Input: part model. Units: mm. Frame: model coordinates. A direction names the side the tool comes from. Coordinates: 2 decimals unless noted, no trailing zeros. Write each loop counter-clockwise with the first axis right and the second up, starting at its lowest first coordinate (ties: lowest second). Pieces come first, ordered by that corner, then holes. Notation, with made-up numbers: (-14, 59.5) - (3, 59.5) arc R16 cw to (3, 73.5) - close; hole circle Ø5 at (-6.5, 88). An arc over 180 degrees is marked (long way). One line per question, with ' | ' between items. Start each with the question number.
1) Section query D-D on x = -15. Return loops of the section in (y, z), and give its area (3 significant figures).
2) First-contact query: P1, Ø2, axis at x = -7, z = 2.5, coming from the +Y side; P2, Ø1.3, axis at x = 4.5, y = 19, coming from the -Z side; P3, Ø1.5, axis at x = 0, z = -0.5, coming from the -Y side; P4, Ø3, axis at y = -8, z = 1, coming from the +X side. Flat tips, straight axial feed; report the tip coordinate or a pass-through.
3) Section query B-B on y = -4.5. Return loops of the section in (x, z).
4) Section query A-A on x = 12.5. Return loops of the section in (y, z), and give its area (3 significant figures).
5) Draft query along Y for faces 4 (the flat face through (0, -15.24, 0)), 5 (the flat face through (-10.16, -17, 0)), 6 (the flat face through (8.924, -7, 0)). Return one class per face: released by +Y, released by -Y, zero draft, split by the parting line, or undercut.
6) Reachability of faces 1 (the flat face through (-19, 9.906, 0)), 2 (the flat face through (0, -17, 2.54)), 3 (the flat face through (3.43, 2.72, 0.07)) from +Z, -Z, +X, -X, +Y, -Y: full face, straight path, thin tool, end or side. Return the list, or none.
7) Line query: line 1 (Y direction, x = 11, z = -2); line 2 (Z direction, x = 15.5, y = 0.5); line 3 (X direction, y = 10, z = 4.75). Output: solid intervals per line, ascending.
8) Section query C-C on x = 8. Return loops of the section in (y, z), and give its area (3 significant figures).
```python
from build123d import *

# Parameters (mm, degrees)
F0_W     = 35.56
F0_H     = 35.56
F1_DEPTH = 5.08
F2_W     = 19.812
F2_H     = 4.572
F3_DEPTH = 2.54
F4_W     = 19.812
F4_H     = 4.572
F5_DEPTH = 2.54
F6_W     = 20.32
F6_H     = 5.08
F7_DEPTH = 2.54
F8_W     = 20.32
F8_H     = 5.08
F9_DEPTH = 2.54


with BuildPart() as f1:
    # F0 (on Top) → F1 (new body, symmetric)
    with BuildSketch(Plane.XY):
        Rectangle(F0_W, F0_H)
        with BuildLine():
            Line((2.5355902778, -12.7), (-2.3592013889, -12.7))
            Line((-2.3592013889, -12.7), (-8.4225694444, 7.0555555556))
            Line((-8.4225694444, 7.0555555556), (-8.5769097222, 7.0555555556))
            add(Edge.make_bspline(
                [(-8.5769097222, 7.0555555556), (-8.2461805556, 1.0307725694), (-8.2461805556, -0.9866753472)],
                knots=[0, 0, 0, 1, 1, 1], degree=2))
            Line((-8.2461805556, -0.9866753472), (-8.2461805556, -12.7))
            Line((-8.2461805556, -12.7), (-13.0197048611, -12.7))
            Line((-13.0197048611, -12.7), (-13.0197048611, 12.4850260417))
            Line((-13.0197048611, 12.4850260417), (-5.7491753472, 12.4850260417))
            Line((-5.7491753472, 12.4850260417), (0.2094618056, -6.7744357639))
            Line((0.2094618056, -6.7744357639), (0.3141927083, -6.7744357639))
            Line((0.3141927083, -6.7744357639), (6.6366319444, 12.4850260417))
            Line((6.6366319444, 12.4850260417), (13.9016493056, 12.4850260417))
            Line((13.9016493056, 12.4850260417), (13.9016493056, -12.7))
            Line((13.9016493056, -12.7), (8.9241753472, -12.7))
            Line((8.9241753472, -12.7), (8.9241753472, -0.7772135417))
            add(Edge.make_bspline(
                [(8.9241753472, -0.7772135417), (8.9241753472, 0.0661458333), (8.9517361111, 1.1685763889)],
                knots=[0, 0, 0, 1, 1, 1], degree=2))
            add(Edge.make_bspline(
                [(8.9517361111, 1.1685763889), (8.979296875, 2.2710069444), (9.1832465278, 7.0224826389)],
                knots=[0, 0, 0, 1, 1, 1], degree=2))
            Line((9.1832465278, 7.0224826389), (9.02890625, 7.0224826389))
            Line((9.02890625, 7.0224826389), (2.5355902778, -12.7))
        make_face(mode=Mode.SUBTRACT)
    extrude(amount=F1_DEPTH, both=True)

    # F2 (on face) → F3 (join)
    with BuildSketch(Plane(origin=(0, 17.78, 0), x_dir=(-1, 0, 0), z_dir=(0, 1, 0))):
        Rectangle(F2_W, F2_H)
    extrude(amount=F3_DEPTH)

    # F4 (on face) → F5 (join)
    with BuildSketch(Plane(origin=(-17.78, 0, 0), x_dir=(0, -1, 0), z_dir=(-1, 0, 0))):
        Rectangle(F4_W, F4_H)
    extrude(amount=F5_DEPTH)

    # F6 (on face) → F7 (cut)
    with BuildSketch(Plane.XZ.offset(17.78)):
        Rectangle(F6_W, F6_H)
    extrude(amount=-F7_DEPTH, mode=Mode.SUBTRACT)

    # F8 (on face) → F9 (cut)
    with BuildSketch(Plane.YZ.offset(17.78)):
        Rectangle(F8_W, F8_H)
    extrude(amount=-F9_DEPTH, mode=Mode.SUBTRACT)


solid = f1.part
```
Answer key:
1) outline: (-17.78, -5.08) - (17.78, -5.08) - (17.78, 5.08) - (-17.78, 5.08) - close | area: 361 mm²
2) P1: y = 20.32 | P2: z = -2.29 | P3: y = -15.24 | P4: x = 15.24
3) outline: (-20.32, -2.29) - (-17.78, -2.29) - (-17.78, -5.08) - (-13.02, -5.08) - (-13.02, 5.08) - (-17.78, 5.08) - (-17.78, 2.29) - (-20.32, 2.29) - close; (-8.25, -5.08) - (-4.88, -5.08) - (-4.88, 5.08) - (-8.25, 5.08) - close; (-0.49, -5.08) - (1.06, -5.08) - (1.06, 5.08) - (-0.49, 5.08) - close; (5.24, -5.08) - (8.92, -5.08) - (8.92, 5.08) - (5.24, 5.08) - close; (13.9, -5.08) - (17.78, -5.08) - (17.78, -2.54) - (15.24, -2.54) - (15.24, 2.54) - (17.78, 2.54) - (17.78, 5.08) - (13.9, 5.08) - close
4) outline: (-17.78, -5.08) - (-12.7, -5.08) - (-12.7, 5.08) - (-17.78, 5.08) - close; (12.49, -5.08) - (17.78, -5.08) - (17.78, 5.08) - (12.49, 5.08) - close | area: 105 mm²
5) face 4: released by -Y | face 5: zero draft | face 6: undercut
6) face 1: +Z, -Z, -X, +Y | face 2: -Y | face 3: +Z, -Z
7) line 1: -17.78 to -12.7, 12.49 to 17.78 | line 2: -5.08 to -2.54, 2.54 to 5.08 | line 3: -17.78 to -13.02, -4.98 to 5.82, 13.9 to 17.78
8) outline: (-17.78, -5.08) - (3.9, -5.08) - (3.9, 5.08) - (-17.78, 5.08) - (-17.78, 2.54) - (-15.24, 2.54) - (-15.24, -2.54) - (-17.78, -2.54) - close; (12.49, -5.08) - (17.78, -5.08) - (17.78, -2.29) - (20.32, -2.29) - (20.32, 2.29) - (17.78, 2.29) - (17.78, 5.08) - (12.49, 5.08) - close | area: 273 mm²
